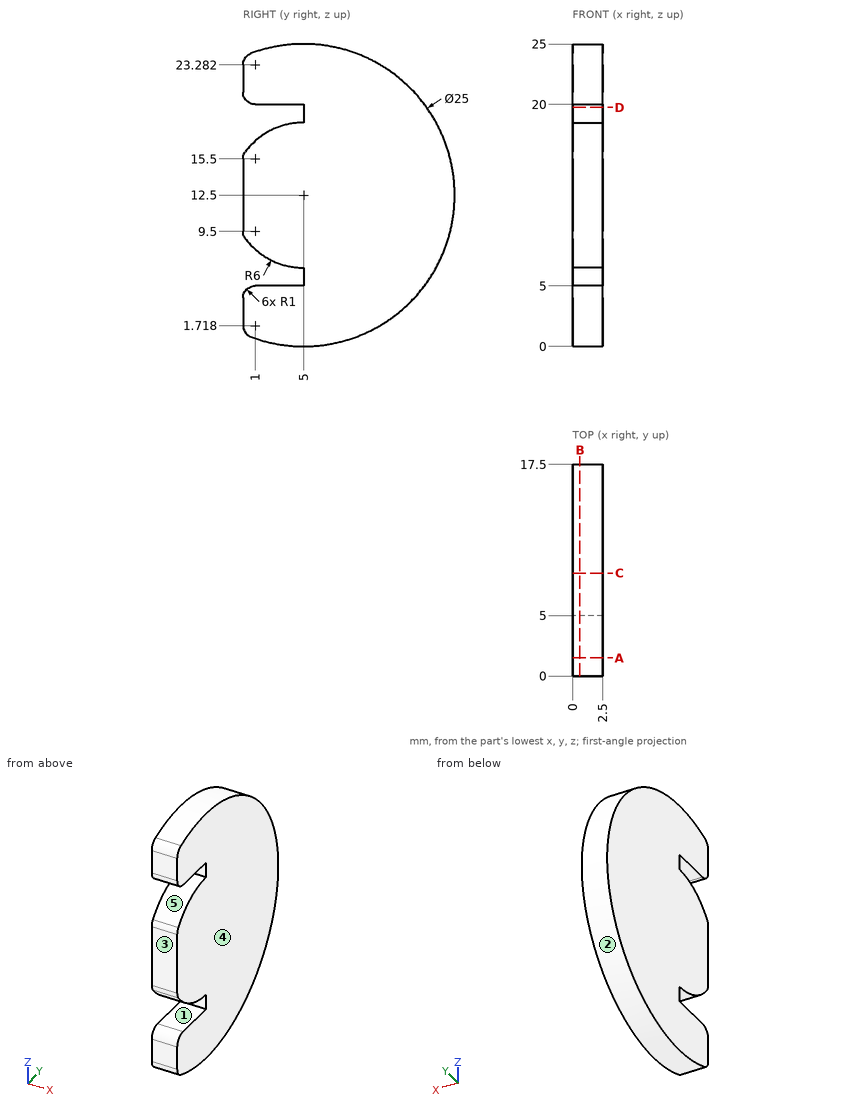
Geometry check sheet. Reference: drawing and pictorial views, mm from the part's lowest x, y, z. A direction names the side the tool comes from. Round coordinates to 2 decimals unless told otherwise and drop trailing zeros. Write each loop counter-clockwise with the first axis right and the second up, starting at its lowest first coordinate (ties: lowest second). Pieces come first, ordered by that corner, then holes. Notation, with made-up numbers: (40, 7) -> (59, 7) arc R31 cw to (59, 39) -> close; hole circle Ø10 at (36.5, -2). An arc over 180 degrees is marked (long way). Answer as CSV lines item,"result". Start each with the question number.
1) Section check A-A on y = 1.5. Enter the section's corners in (x, z), and give its area (3 significant figures).
2) Tool access check on the marked faces 4 and 5. Record the directions out of +Z, -Z, +X, -X, +Y, -Y that give a thin tool (end or side, any length) a straight path to the whole face; none if there is none.
3) Material ranges on line 1 (Z direction, x = 0.4, y = 2); line 2 (Z direction, x = 0.55, y = 1.75); line 3 (Z direction, x = 1.45, y = 9.5), recorded low to high. Write a range as from..to.
4) Go/stop test with flat-tipped pins: P1, Ø1.5, axis at x = 1, y = 11, coming from the -Z side; P2, Ø1, axis at x = 1.5, y = 15, coming from the +Z side. Record where each tip stops, or that it passes through.
5) Release check for a two-part mould opening along Z. For the marked faces 1, 2 and 3 record: pulls with the +Z half, pulls with the -Z half, needs draft (parallel to the pull), parting line crosses it, or undercut.
6) Section check D-D on z = 19.75. Enter the section's corners in (x, y), and give its area (3 significant figures).
7) Section check B-B on x = 0.6. Enter the section's corners in (y, z), and give its area (3 significant figures).
8) Section check C-C on y = 8.5. Enter the section's corners in (x, z).
Found:
1,outline,"(0, 0.5) -> (2.5, 0.5) -> (2.5, 5) -> (0, 5) -> close; (0, 7.63) -> (2.5, 7.63) -> (2.5, 17.37) -> (0, 17.37) -> close; (0, 20) -> (2.5, 20) -> (2.5, 24.5) -> (0, 24.5) -> close"
1,area,"46.9 mm^2"
2,face 4,"+Z, -Z, +X, +Y, -Y"
2,face 5,"+X, -X, -Y"
3,line 1,"z = 0.37..5, 7.3..17.7, 20..24.63"
3,line 2,"z = 0.43..5, 7.46..17.54, 20..24.57"
3,line 3,"z = 0.84..24.16"
4,P1,"stops at z = 1.16"
4,P2,"stops at z = 20.62"
5,face 1,"undercut"
5,face 2,"parting line crosses it"
5,face 3,"needs draft"
6,outline,"(0, 5) -> (2.5, 5) -> (2.5, 15.18) -> (0, 15.18) -> close"
6,area,"25.5 mm^2"
7,outline,"(0, 1.72) arc R1 ccw to (0.65, 0.78) arc R12.5 ccw (long way) to (0.65, 24.22) arc R1 ccw to (0, 23.28) -> (0, 21) arc R1 ccw to (1, 20) -> (5, 20) -> (5, 18.5) arc R6 ccw to (0.2, 16.1) arc R1 ccw to (0, 15.5) -> (0, 9.5) arc R1 ccw to (0.2, 8.9) arc R6 ccw to (5, 6.5) -> (5, 5) -> (1, 5) arc R1 ccw to (0, 4) -> close"
7,area,"343 mm^2"
8,outline,"(0, 0.5) -> (2.5, 0.5) -> (2.5, 24.5) -> (0, 24.5) -> close"
